from build123d import *

# Parameters (mm, degrees)
F0_R     = 44.45
F0_R_2   = 12.7
F1_DEPTH = 25.4


with BuildPart() as f1:
    # F0 (on Front) → F1 (new body)
    with BuildSketch(Plane.XZ):
        with BuildLine():
            Line((-46.08459, -48.703328), (-46.08459, -58.516014))
            Line((-46.08459, -58.516014), (46.08459, -58.516014))
            Line((46.08459, -58.516014), (46.08459, -48.703328))
            ThreePointArc((46.08459, -48.703328), (47.944462, -44.2132), (52.43459, -42.353328))
            Line((52.43459, -42.353328), (65.728895, -42.353328))
            Line((65.728895, -42.353328), (65.728895, 54.819994))
            Line((65.728895, 54.819994), (42.319705, 54.819994))
            ThreePointArc((42.319705, 54.819994), (27.951295, 60.771584), (21.999705, 75.139994))
            Line((21.999705, 75.139994), (21.999705, 327.922707))
            Line((21.999705, 327.922707), (50.8, 327.922707))
            Line((50.8, 327.922707), (50.8, 392.02783))
            Line((50.8, 392.02783), (-50.8, 392.02783))
            Line((-50.8, 392.02783), (-50.8, 327.922707))
            Line((-50.8, 327.922707), (-21.999705, 327.922707))
            Line((-21.999705, 327.922707), (-21.999705, 321.452414))
            Line((-21.999705, 321.452414), (-21.999705, 73.922707))
            ThreePointArc((-21.999705, 73.922707), (-27.951295, 59.554297), (-42.319705, 53.602707))
            Line((-42.319705, 53.602707), (-65.728895, 53.602707))
            Line((-65.728895, 53.602707), (-65.728895, -42.353328))
            Line((-65.728895, -42.353328), (-52.43459, -42.353328))
            ThreePointArc((-52.43459, -42.353328), (-47.944462, -44.2132), (-46.08459, -48.703328))
        make_face()
        Circle(F0_R, mode=Mode.SUBTRACT)
        with Locations((0, 356.401086)):
            Circle(F0_R_2, mode=Mode.SUBTRACT)
    extrude(amount=F1_DEPTH)


solid = f1.part
Could you check a few things on this model? Use its own coordinates, in mm. A direction names the side the tool comes from. Give positions to 0.01 mm unless a question says otherwise; leave off trailing zeros. Order: outer loops, then holes, each group sorted by start corner. A loop starts at its lowest first (then second) coordinate and runs counter-clockwise, first axis right, second up.
1. I need wall thicknesses on L1, parallel to Z at x = 0, y = -6.5; L2, parallel to Z at x = 40, y = -15.75; L3, parallel to X at y = -7, z = 313.5. Which ranges of each line are inside material? Lowest first, please.
2. Suppose I cut it at D-D (x = 0). List the corners of the cut face in (y, z) for me, plus the area to 3 significant figures.
3. Suppose I cut it at A-A (z = 0). List the corners of the cut face in (x, y) for me, plus the area to 3 significant figures.
4. For faces 1 (the flat face through (50.8, -13, 360)), 2 (the flat face through (59, -13, -42.353)), 3 (the cylindrical face through (-27.794, -12.522, 59.713)), 4 (the flat face through (-50.8, -13, 360)), which set-ups out of +Z, -Z, +X, -X, +Y, -Y let a thin tool reach every point of the face, with its end or its side?
5. Suppose I cut it at C-C (y = -14.5). List the corners of the cut face in (x, z) for me, plus the area to 3 significant figures.
6. Suppose I cut it at B-B (x = -38.5). List the corners of the cut face in (y, z) for me.
7. We'd pull the mould along X, two halves only. Please class faces 5 (the cylindrical face through (28.11, -12.522, 60.614)), 6 (the flat face through (36, -13, 327.923)), 7 (the cylindrical face through (42.397, -12.522, 13.352)): pulls with the +X half, pulls with the -X half, needs draft (parallel to the pull), parting line crosses it, or undercut.
8. Will these pins go through, and if not, where does the flat tip stop? P1, Ø5, axis at y = -17, z = -55, coming from the -X side; P2, Ø4, axis at y = -8, z = 261, coming from the +X side; P3, Ø14.5, axis at x = -62, y = -7.5, coming from the -Z side.
Solved:
1. L1: z = -58.52 to -44.45, 44.45 to 343.7, 369.1 to 392.03
1. L2: z = -58.52 to -19.39, 19.39 to 54.95, 327.92 to 392.03
1. L3: x = -22 to 22
2. outline: (-25.4, -58.52) - (0, -58.52) - (0, -44.45) - (-25.4, -44.45) - close; (-25.4, 44.45) - (0, 44.45) - (0, 343.7) - (-25.4, 343.7) - close; (-25.4, 369.1) - (0, 369.1) - (0, 392.03) - (-25.4, 392.03) - close
2. area: 8,540 mm2
3. outline: (-65.73, -25.4) - (-44.45, -25.4) - (-44.45, 0) - (-65.73, 0) - close; (44.45, -25.4) - (65.73, -25.4) - (65.73, 0) - (44.45, 0) - close
3. area: 1,080 mm2
4. face 1: +Z, +X, +Y, -Y
4. face 2: -Z, +X, +Y, -Y
4. face 3: -X, +Y, -Y
4. face 4: +Z, -X, +Y, -Y
5. outline: (-65.73, -42.35) - (-52.43, -42.35) arc R6.35 cw to (-46.08, -48.7) - (-46.08, -58.52) - (46.08, -58.52) - (46.08, -48.7) arc R6.35 cw to (52.43, -42.35) - (65.73, -42.35) - (65.73, 54.82) - (42.32, 54.82) arc R20.32 cw to (22, 75.14) - (22, 327.92) - (50.8, 327.92) - (50.8, 392.03) - (-50.8, 392.03) - (-50.8, 327.92) - (-22, 327.92) - (-22, 73.92) arc R20.32 cw to (-42.32, 53.6) - (-65.73, 53.6) - close; hole circle Ø88.9 at (0, 0); hole circle Ø25.4 at (0, 356.4)
5. area: 26,200 mm2
6. outline: (-25.4, -58.52) - (0, -58.52) - (0, -22.22) - (-25.4, -22.22) - close; (-25.4, 22.22) - (0, 22.22) - (0, 53.96) - (-25.4, 53.96) - close; (-25.4, 327.92) - (0, 327.92) - (0, 392.03) - (-25.4, 392.03) - close
7. face 5: pulls with the +X half
7. face 6: needs draft
7. face 7: undercut
8. P1: stops at x = -46.08
8. P2: stops at x = 22
8. P3: stops at z = -42.35
